Check sheet for the modelled part. Datum: model origin and axes. Units: mm. Give positions to 0.01 mm unless a question says otherwise; leave off trailing zeros. Order: outer loops, then holes, each group sorted by start corner. A loop starts at its lowest first (then second) coordinate and runs counter-clockwise, first axis right, second up. Notation, with made-up numbers: (24.5, 48) -> (51.5, 48) arc R32 ccw to (51.5, 76) -> close; hole circle Ø3 at (-13.75, 49). An arc over 180 degrees is marked (long way). One line per question, with ' | ' between items.
```python
from build123d import *

# Parameters (mm, degrees)
SKETCH1_R           = 15
SKETCH1_R_2         = 1.5
BOSS_EXTRUDE1_DEPTH = 2
FILLET1_R           = 2


with BuildPart() as part:
    # Sketch1 → Boss-Extrude1 (new body)
    with BuildSketch(Plane.XY):
        with BuildLine():
            Line((-22.557559524, -19.777677021), (-4.949747468, -19.777677021))
            ThreePointArc((-4.949747468, -19.777677021), (-3.181980515, -19.045443974), (-2.449747468, -17.277677021))
            Line((-2.449747468, -17.277677021), (17.277677021, 2.449747468))
            ThreePointArc((17.277677021, 2.449747468), (19.045443974, 3.181980515), (19.777677021, 4.949747468))
            Line((19.777677021, 4.949747468), (19.777677021, 22.557559524))
            ThreePointArc((19.777677021, 22.557559524), (-21.213203436, 21.213203436), (-22.557559524, -19.777677021))
        make_face()
        with Locations((-4.949747468, 4.949747468)):
            Circle(SKETCH1_R, mode=Mode.SUBTRACT)
        with Locations((-4.949747468, -17.277677021)):
            Circle(SKETCH1_R_2, mode=Mode.SUBTRACT)
        with Locations((17.277677021, 4.949747468)):
            Circle(SKETCH1_R_2, mode=Mode.SUBTRACT)
    extrude(amount=BOSS_EXTRUDE1_DEPTH)

    # Fillet1
    fillet1_edges = [part.edges().sort_by_distance(p)[0] for p in [
        (-22.557559524, -19.777677021, 1),
        (19.777677021, 22.557559524, 1),
    ]]
    fillet(fillet1_edges, radius=FILLET1_R)


solid = part.part
```
Q1. Depth check by flat-ended pin: pin 1 Ø6 at (x, y) = (8.5, 0) entering from +Z. Enter the tip coordinate at first touch or a pass-through.
Result sheet:
pin 1: stops at z = 2
Q2. Section check B-B (x = -15). Enter the section's corners in (y, z).
Result sheet:
outline: (-19.78, 0) -> (-6.19, 0) -> (-6.19, 2) -> (-19.78, 2) -> close; (16.08, 0) -> (25.98, 0) -> (25.98, 2) -> (16.08, 2) -> close
Q3. Section check C-C (y = -2). Enter the section's corners in (x, z), and give its area (3 significant figures).
Result sheet:
outline: (-29.93, 0) -> (-18.24, 0) -> (-18.24, 2) -> (-29.93, 2) -> close; (8.34, 0) -> (12.83, 0) -> (12.83, 2) -> (8.34, 2) -> close | area: 32.4 mm2
Q4. Thickness scan on line 1 (X direction, y = -7, z = 0.55); line 2 (X direction, y = 8, z = 1.8); line 3 (X direction, y = 6, z = 1.6). Record the ranges inside material, lowest first.
Result sheet:
line 1: x = -29.17 to -14.02, 4.12 to 7.83 | line 2: x = -28.91 to -19.64, 9.74 to 19.78 | line 3: x = -29.39 to -19.91, 10.01 to 16.21, 18.35 to 19.78
Q5. Section check A-A (z = 0.3). Enter the section's corners in (x, y).
Result sheet:
outline: (-23.18, -19.05) arc R2 ccw to (-21.63, -19.78) -> (-4.95, -19.78) arc R2.5 ccw to (-2.45, -17.28) -> (17.28, 2.45) arc R2.5 ccw to (19.78, 4.95) -> (19.78, 21.63) arc R2 ccw to (19.05, 23.18) arc R30 ccw to start; hole circle Ø30 at (-4.95, 4.95); hole circle Ø3 at (-4.95, -17.28); hole circle Ø3 at (17.28, 4.95)
Q6. Mould release check, pull along X, two halves, no side actions. Record for faces 1 (the face through (7.28, -7.55, 0.99)), 2 (the face through (-17, 17, 0)), 3 (the face through (-5.275, -18.742, 0.986)): pulls with the +X half, pulls with the -X half, needs draft (parallel to the pull), parting line crosses it, or undercut.
Result sheet:
face 1: pulls with the +X half | face 2: needs draft | face 3: undercut
Q7. Section check D-D (y = 26). Enter the section's corners in (x, z).
Result sheet:
outline: (-14.97, 0) -> (14.97, 0) -> (14.97, 2) -> (-14.97, 2) -> close
